```python
from build123d import *

# Parameters (mm, degrees)
SKETCH_1_W               = 55
SKETCH_1_H               = 46.3
EXTRUDE_1_DEPTH          = 15
SKETCH_2_W               = 5.6
SKETCH_2_H               = 5.6
CUT_EXTRUDE_1_DEPTH      = 14
SKETCH_3_R               = 1.5
CUT_EXTRUDE_2_DEPTH      = 1
MIRROR_2_COPY_1_SKETCH_W = 5.6
MIRROR_2_COPY_1_SKETCH_H = 5.6
MIRROR_2_COPY_1_DEPTH    = 14
MIRROR_2_COPY_2_SKETCH_R = 1.5
MIRROR_2_COPY_2_DEPTH    = 1
FILLET_1_R               = 3
FILLET_2_R               = 0.8
SKETCH_5_W               = 4
SKETCH_5_H               = 36
EXTRUDE_2_DEPTH          = 5.5
SKETCH_6_R               = 1.5
EXTRUDE_3_DEPTH          = 1.5
SKETCH_7_W               = 36
SKETCH_7_H               = 9
SKETCH_7_W_2             = 34
SKETCH_7_H_2             = 7
SKETCH_7_W_3             = 7
SKETCH_7_H_3             = 13
SKETCH_7_W_4             = 5
SKETCH_7_H_4             = 11
EXTRUDE_4_DEPTH          = 10
SKETCH_9_W               = 34
SKETCH_9_H               = 8
CUT_EXTRUDE_3_DEPTH      = 11


with BuildPart() as part:
    # 草图1 → 凸台-拉伸1 (new body)
    with BuildSketch(Plane.XY):
        Rectangle(SKETCH_1_W, SKETCH_1_H)
    extrude(amount=EXTRUDE_1_DEPTH)

    # 草图2 → 切除-拉伸1 (cut)
    with BuildSketch(Plane.XY.offset(15)):
        with Locations((-24.7, 20.35)):
            Rectangle(SKETCH_2_W, SKETCH_2_H)
    cut_extrude_1 = extrude(amount=-CUT_EXTRUDE_1_DEPTH, mode=Mode.SUBTRACT)

    # 草图3 → 切除-拉伸2 (cut)
    with BuildSketch(Plane.XY.offset(1)):
        with Locations((-24.7, 20.35)):
            Circle(SKETCH_3_R)
    cut_extrude_2 = extrude(amount=-CUT_EXTRUDE_2_DEPTH, mode=Mode.SUBTRACT)

    # 镜向1: 切除-拉伸1, 切除-拉伸2 across plane
    add(cut_extrude_1.mirror(Plane.ZX), mode=Mode.SUBTRACT)
    add(cut_extrude_2.mirror(Plane.ZX), mode=Mode.SUBTRACT)

    # 镜向2: 切除-拉伸1, 切除-拉伸2 across plane
    add(cut_extrude_1.mirror(Plane(origin=(0, 0, 0), x_dir=(0, 0, 1), z_dir=(1, 0, 0))), mode=Mode.SUBTRACT)
    add(cut_extrude_2.mirror(Plane(origin=(0, 0, 0), x_dir=(0, 0, 1), z_dir=(1, 0, 0))), mode=Mode.SUBTRACT)

    # 镜向2 copy 1 sketch → 镜向2 copy 1 (cut)
    with BuildSketch(Plane(origin=(0, 0, 15), x_dir=(-1, 0, 0), z_dir=(0, 0, 1))):
        with Locations((-24.7, 20.35)):
            Rectangle(MIRROR_2_COPY_1_SKETCH_W, MIRROR_2_COPY_1_SKETCH_H)
    extrude(amount=-MIRROR_2_COPY_1_DEPTH, mode=Mode.SUBTRACT)

    # 镜向2 copy 2 sketch → 镜向2 copy 2 (cut)
    with BuildSketch(Plane(origin=(0, 0, 1), x_dir=(-1, 0, 0), z_dir=(0, 0, 1))):
        with Locations((-24.7, 20.35)):
            Circle(MIRROR_2_COPY_2_SKETCH_R)
    extrude(amount=-MIRROR_2_COPY_2_DEPTH, mode=Mode.SUBTRACT)

    # 圆角1
    fillet_1_edges = [part.edges().sort_by_distance(p)[0] for p in [
        (-27.5, 23.15, 0.5),
        (-27.5, -23.15, 0.5),
        (27.5, -23.15, 0.5),
        (27.5, 23.15, 0.5),
    ]]
    fillet(fillet_1_edges, radius=FILLET_1_R)

    # 圆角2
    fillet_2_edges = [part.edges().sort_by_distance(p)[0] for p in [
        (-27.5, 0, 15),
        (-27.5, 17.55, 8),
        (-21.9, 23.15, 8),
        (-21.9, 17.55, 8),
        (-24.7, 17.55, 15),
        (-21.9, 20.35, 15),
        (0, -23.15, 15),
        (-24.7, -17.55, 15),
        (-27.5, -17.55, 8),
        (-21.9, -20.35, 15),
        (-21.9, -17.55, 8),
        (-21.9, -23.15, 8),
        (27.5, 0, 15),
        (27.5, -17.55, 8),
        (21.9, -23.15, 8),
        (21.9, -17.55, 8),
        (24.7, -17.55, 15),
        (21.9, -20.35, 15),
        (0, 23.15, 15),
        (24.7, 17.55, 15),
        (27.5, 17.55, 8),
        (21.9, 20.35, 15),
        (21.9, 17.55, 8),
        (21.9, 23.15, 8),
    ]]
    fillet(fillet_2_edges, radius=FILLET_2_R)

    # 草图5 → 凸台-拉伸2 (add)
    with BuildSketch(Plane.XY.offset(15)):
        with Locations((-13, 0)):
            Rectangle(SKETCH_5_W, SKETCH_5_H)
        with Locations((13, 0)):
            Rectangle(SKETCH_5_W, SKETCH_5_H)
    extrude(amount=EXTRUDE_2_DEPTH)

    # 草图6 → 凸台-拉伸3 (add)
    with BuildSketch(Plane.XY.offset(20.5)):
        with BuildLine():
            Line((24.5, 23.15), (-24.5, 23.15))
            ThreePointArc((-24.5, 23.15), (-26.621320344, 22.271320344), (-27.5, 20.15))
            Line((-27.5, 20.15), (-27.5, -20.15))
            ThreePointArc((-27.5, -20.15), (-26.621320344, -22.271320344), (-24.5, -23.15))
            Line((-24.5, -23.15), (24.5, -23.15))
            ThreePointArc((24.5, -23.15), (26.621320344, -22.271320344), (27.5, -20.15))
            Line((27.5, -20.15), (27.5, 20.15))
            ThreePointArc((27.5, 20.15), (26.621320344, 22.271320344), (24.5, 23.15))
        make_face()
        with Locations((-24.7, 20.35)):
            Circle(SKETCH_6_R, mode=Mode.SUBTRACT)
        with Locations((24.7, 20.35)):
            Circle(SKETCH_6_R, mode=Mode.SUBTRACT)
        with Locations((-24.7, -20.35)):
            Circle(SKETCH_6_R, mode=Mode.SUBTRACT)
        with Locations((24.7, -20.35)):
            Circle(SKETCH_6_R, mode=Mode.SUBTRACT)
    extrude(amount=EXTRUDE_3_DEPTH)

    # 草图7 → 凸台-拉伸4 (add)
    with BuildSketch(Plane.XY.offset(22)):
        with Locations((3.5, 18.65)):
            Rectangle(SKETCH_7_W, SKETCH_7_H)
        with Locations((3.5, 18.65)):
            Rectangle(SKETCH_7_W_2, SKETCH_7_H_2, mode=Mode.SUBTRACT)
        with Locations((10, 4.65)):
            Rectangle(SKETCH_7_W_3, SKETCH_7_H_3)
        with Locations((10, 4.65)):
            Rectangle(SKETCH_7_W_4, SKETCH_7_H_4, mode=Mode.SUBTRACT)
        with Locations((-3, -16.65)):
            Rectangle(SKETCH_7_W, SKETCH_7_H_3)
    extrude(amount=EXTRUDE_4_DEPTH)

    # 草图9 → 切除-拉伸3 (cut)
    with BuildSketch(Plane.XZ.offset(23.15)):
        with Locations((-3, 27)):
            Rectangle(SKETCH_9_W, SKETCH_9_H)
    extrude(amount=-CUT_EXTRUDE_3_DEPTH, mode=Mode.SUBTRACT)


solid = part.part
```
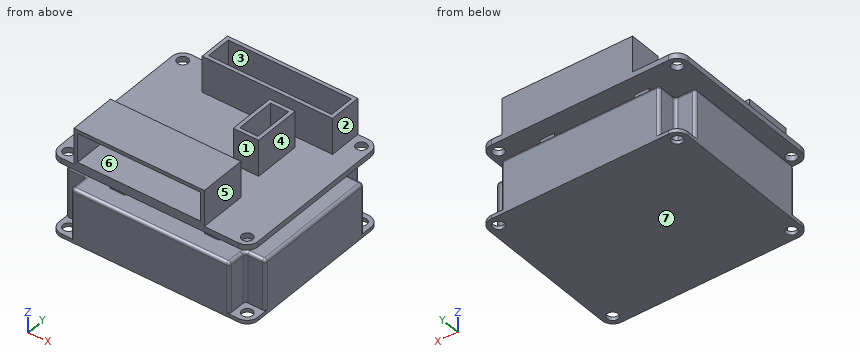
Here's how the part is built. I have some questions about the finished solid (model axes, mm). Face numbers are marked on the shaded views. A direction names the side the tool comes from. Round coordinates to 2 decimals unless told otherwise and drop trailing zeros. Loops run counter-clockwise (first coordinate to the right, second up) from the corner with the lowest first, then second, coordinate; pieces in that order, holes last.
1. Suppose I cut it at C-C, the plane z = 10. Please give me the cut outline in (x, y).
Answers:
outline: (-27.5, -16.75) arc R0.8 ccw to (-26.7, -17.55) - (-22.7, -17.55) arc R0.8 cw to (-21.9, -18.35) - (-21.9, -22.35) arc R0.8 ccw to (-21.1, -23.15) - (21.1, -23.15) arc R0.8 ccw to (21.9, -22.35) - (21.9, -18.35) arc R0.8 cw to (22.7, -17.55) - (26.7, -17.55) arc R0.8 ccw to (27.5, -16.75) - (27.5, 16.75) arc R0.8 ccw to (26.7, 17.55) - (22.7, 17.55) arc R0.8 cw to (21.9, 18.35) - (21.9, 22.35) arc R0.8 ccw to (21.1, 23.15) - (-21.1, 23.15) arc R0.8 ccw to (-21.9, 22.35) - (-21.9, 18.35) arc R0.8 cw to (-22.7, 17.55) - (-26.7, 17.55) arc R0.8 ccw to (-27.5, 16.75) - close
2. For the marked faces 1, 2, 3 and 4, which set-ups out of +Z, -Z, +X, -X, +Y, -Y let a thin tool reach every point of the face, with its end or its side?
Answers:
face 1: +Z, +X, -X
face 2: +Z, +X, +Y, -Y
face 3: +Z
face 4: +Z, +X
3. Suppose I cut it at B-B, the plane y = -9.5. Please give me the cut outline in (x, z).
Answers:
outline: (-27.5, 0) - (27.5, 0) - (27.5, 14.2) arc R0.8 ccw to (26.7, 15) - (15, 15) - (15, 20.5) - (27.5, 20.5) - (27.5, 22) - (-27.5, 22) - (-27.5, 20.5) - (-15, 20.5) - (-15, 15) - (-26.7, 15) arc R0.8 ccw to (-27.5, 14.2) - close; hole (-11, 15) - (11, 15) - (11, 20.5) - (-11, 20.5) - close
4. Suppose I cut it at A-A, the plane x = 2. Please give me the cut outline in (y, z), and give its area (3 significant figures).
Answers:
outline: (-23.15, 0) - (23.15, 0) - (23.15, 14.2) arc R0.8 ccw to (22.35, 15) - (-22.35, 15) arc R0.8 ccw to (-23.15, 14.2) - close; (-23.15, 20.5) - (23.15, 20.5) - (23.15, 32) - (22.15, 32) - (22.15, 22) - (15.15, 22) - (15.15, 32) - (14.15, 32) - (14.15, 22) - (-10.15, 22) - (-10.15, 32) - (-23.15, 32) - (-23.15, 31) - (-12.15, 31) - (-12.15, 23) - (-23.15, 23) - close
area: 826 mm2
5. Suppose I cut it at D-D, the plane y = 0. Please give me the cut outline in (x, z).
Answers:
outline: (-27.5, 0) - (27.5, 0) - (27.5, 14.2) arc R0.8 ccw to (26.7, 15) - (15, 15) - (15, 20.5) - (27.5, 20.5) - (27.5, 22) - (13.5, 22) - (13.5, 32) - (12.5, 32) - (12.5, 22) - (7.5, 22) - (7.5, 32) - (6.5, 32) - (6.5, 22) - (-27.5, 22) - (-27.5, 20.5) - (-15, 20.5) - (-15, 15) - (-26.7, 15) arc R0.8 ccw to (-27.5, 14.2) - close; hole (-11, 15) - (11, 15) - (11, 20.5) - (-11, 20.5) - close
6. Thinking about a two-plate mould opening in Z: for the marked faces 5, 6 and 7, which applies, released by +Z, released by -Z, zero draft, split by the parting line, or undercut?
Answers:
face 5: zero draft
face 6: undercut
face 7: released by -Z
7. Will these pins go through, and if not, where does the flat tip stop? pin 1 (4 mm diameter, centred on y = 1, z = 16.5, fed in from -X); pin 2 (1.2 mm diameter, centred on y = -19.5, z = 9, fed in from +X); pin 3 (5.5 mm diameter, centred on x = 11, z = 29, fed in from -Y); pin 4 (2 mm diameter, centred on y = 11.5, z = 23.5, fed in from +X).
Answers:
pin 1: stops at x = -27.44
pin 2: stops at x = 21.9
pin 3: stops at y = -23.15
pin 4: stops at x = 13.5
8. If I drill on probe 1 along Y at (x, z) = (24.7, 21.5); probe 2 along Z at (x, y) = (-6.5, -21); probe 3 along Z at (x, y) = (22, 19), over which ranges is the centre line in solid material (lowest first)?
Answers:
probe 1: y = -23.14 to -21.85, -18.85 to 18.85, 21.85 to 23.14
probe 2: z = 0 to 15, 20.5 to 23, 31 to 32
probe 3: z = 0 to 1, 20.5 to 22
